Model file for the job. Use its own axes, mm. A direction names the side the tool comes from. Give positions to 0.01 mm unless a question says otherwise; leave off trailing zeros. Loops run counter-clockwise (first coordinate to the right, second up) from the corner with the lowest first, then second, coordinate; pieces in that order, holes last. Notation, with made-up numbers: (29.5, -19) - (87.5, -19) arc R5 cw to (87.5, -15) - close; hole circle Ø9 at (33.5, -8). An arc over 180 degrees is marked (long way). Use a Markdown table: item, result.
from build123d import *

# Parameters (mm, degrees)
SKETCH2_W           = 25
SKETCH2_H           = 25
BOSS_EXTRUDE1_DEPTH = 8
SKETCH5_R           = 0.7
CUT_EXTRUDE2_DEPTH  = 8
SKETCH2_6_W         = 25
SKETCH2_6_H         = 25
SKETCH2_6_W_2       = 20
SKETCH2_6_H_2       = 20
BOSS_EXTRUDE2_DEPTH = 43


with BuildPart() as part:
    # Sketch2 → Boss-Extrude1 (new body)
    with BuildSketch(Plane.XY.offset(43)):
        Rectangle(SKETCH2_W, SKETCH2_H)
    extrude(amount=BOSS_EXTRUDE1_DEPTH)

    # Sketch5 → Cut-Extrude2 (cut)
    with BuildSketch(Plane.XY.offset(43)):
        with Locations((-8.388056057, 8.509622087)):
            Circle(SKETCH5_R)
        with Locations((-6.038056057, 8.509622087)):
            Circle(SKETCH5_R)
        with Locations((-3.688056057, 8.509622087)):
            Circle(SKETCH5_R)
        with Locations((-1.338056057, 8.509622087)):
            Circle(SKETCH5_R)
        with Locations((1.011943943, 8.509622087)):
            Circle(SKETCH5_R)
        with Locations((3.361943943, 8.509622087)):
            Circle(SKETCH5_R)
        with Locations((5.711943943, 8.509622087)):
            Circle(SKETCH5_R)
        with Locations((8.061943943, 8.509622087)):
            Circle(SKETCH5_R)
        with Locations((-6.038056057, 6.159622087)):
            Circle(SKETCH5_R)
        with Locations((-3.688056057, 6.159622087)):
            Circle(SKETCH5_R)
        with Locations((-1.338056057, 6.159622087)):
            Circle(SKETCH5_R)
        with Locations((1.011943943, 6.159622087)):
            Circle(SKETCH5_R)
        with Locations((3.361943943, 6.159622087)):
            Circle(SKETCH5_R)
        with Locations((5.711943943, 6.159622087)):
            Circle(SKETCH5_R)
        with Locations((8.061943943, 6.159622087)):
            Circle(SKETCH5_R)
        with Locations((-6.038056057, 3.809622087)):
            Circle(SKETCH5_R)
        with Locations((-3.688056057, 3.809622087)):
            Circle(SKETCH5_R)
        with Locations((-1.338056057, 3.809622087)):
            Circle(SKETCH5_R)
        with Locations((1.011943943, 3.809622087)):
            Circle(SKETCH5_R)
        with Locations((3.361943943, 3.809622087)):
            Circle(SKETCH5_R)
        with Locations((5.711943943, 3.809622087)):
            Circle(SKETCH5_R)
        with Locations((8.061943943, 3.809622087)):
            Circle(SKETCH5_R)
        with Locations((-6.038056057, 1.459622087)):
            Circle(SKETCH5_R)
        with Locations((-3.688056057, 1.459622087)):
            Circle(SKETCH5_R)
        with Locations((-1.338056057, 1.459622087)):
            Circle(SKETCH5_R)
        with Locations((1.011943943, 1.459622087)):
            Circle(SKETCH5_R)
        with Locations((3.361943943, 1.459622087)):
            Circle(SKETCH5_R)
        with Locations((5.711943943, 1.459622087)):
            Circle(SKETCH5_R)
        with Locations((8.061943943, 1.459622087)):
            Circle(SKETCH5_R)
        with Locations((-6.038056057, -0.890377913)):
            Circle(SKETCH5_R)
        with Locations((-3.688056057, -0.890377913)):
            Circle(SKETCH5_R)
        with Locations((-1.338056057, -0.890377913)):
            Circle(SKETCH5_R)
        with Locations((1.011943943, -0.890377913)):
            Circle(SKETCH5_R)
        with Locations((3.361943943, -0.890377913)):
            Circle(SKETCH5_R)
        with Locations((5.711943943, -0.890377913)):
            Circle(SKETCH5_R)
        with Locations((8.061943943, -0.890377913)):
            Circle(SKETCH5_R)
        with Locations((-6.038056057, -3.240377913)):
            Circle(SKETCH5_R)
        with Locations((-3.688056057, -3.240377913)):
            Circle(SKETCH5_R)
        with Locations((-1.338056057, -3.240377913)):
            Circle(SKETCH5_R)
        with Locations((1.011943943, -3.240377913)):
            Circle(SKETCH5_R)
        with Locations((3.361943943, -3.240377913)):
            Circle(SKETCH5_R)
        with Locations((5.711943943, -3.240377913)):
            Circle(SKETCH5_R)
        with Locations((8.061943943, -3.240377913)):
            Circle(SKETCH5_R)
        with Locations((-6.038056057, -5.590377913)):
            Circle(SKETCH5_R)
        with Locations((-3.688056057, -5.590377913)):
            Circle(SKETCH5_R)
        with Locations((-1.338056057, -5.590377913)):
            Circle(SKETCH5_R)
        with Locations((1.011943943, -5.590377913)):
            Circle(SKETCH5_R)
        with Locations((3.361943943, -5.590377913)):
            Circle(SKETCH5_R)
        with Locations((5.711943943, -5.590377913)):
            Circle(SKETCH5_R)
        with Locations((8.061943943, -5.590377913)):
            Circle(SKETCH5_R)
        with Locations((-6.038056057, -7.940377913)):
            Circle(SKETCH5_R)
        with Locations((-3.688056057, -7.940377913)):
            Circle(SKETCH5_R)
        with Locations((-1.338056057, -7.940377913)):
            Circle(SKETCH5_R)
        with Locations((1.011943943, -7.940377913)):
            Circle(SKETCH5_R)
        with Locations((3.361943943, -7.940377913)):
            Circle(SKETCH5_R)
        with Locations((5.711943943, -7.940377913)):
            Circle(SKETCH5_R)
        with Locations((8.061943943, -7.940377913)):
            Circle(SKETCH5_R)
        with Locations((-8.388056057, 6.159622087)):
            Circle(SKETCH5_R)
        with Locations((-8.388056057, 3.809622087)):
            Circle(SKETCH5_R)
        with Locations((-8.388056057, 1.459622087)):
            Circle(SKETCH5_R)
        with Locations((-8.388056057, -0.890377913)):
            Circle(SKETCH5_R)
        with Locations((-8.388056057, -3.240377913)):
            Circle(SKETCH5_R)
        with Locations((-8.388056057, -5.590377913)):
            Circle(SKETCH5_R)
        with Locations((-8.388056057, -7.940377913)):
            Circle(SKETCH5_R)
    extrude(amount=CUT_EXTRUDE2_DEPTH, mode=Mode.SUBTRACT)

    # Sketch2<6> → Boss-Extrude2 (add)
    with BuildSketch(Plane.XY.offset(43)):
        Rectangle(SKETCH2_6_W, SKETCH2_6_H)
        Rectangle(SKETCH2_6_W_2, SKETCH2_6_H_2, mode=Mode.SUBTRACT)
    extrude(amount=-BOSS_EXTRUDE2_DEPTH)


solid = part.part
(1) Pin check, flat tips, straight feed: P1, Ø1.3, axis at x = -3.69, y = 8.51, coming from the +Z side; P2, Ø12, axis at x = 0.5, y = -2, coming from the -Z side. Stop position of each tip, or through.
Computed:
| item | result |
|---|---|
| P1 | through |
| P2 | z = 43 |
(2) Slice it at A-A, the plane z = 24.5. Write the cut outline in (x, y).
Computed:
| item | result |
|---|---|
| outline | (-12.5, -12.5) - (12.5, -12.5) - (12.5, 12.5) - (-12.5, 12.5) - close; hole (-10, -10) - (10, -10) - (10, 10) - (-10, 10) - close |
(3) Drill centre lines: probe 1 along X at (y, z) = (6.75, 22); probe 2 along Z at (x, y) = (4.25, 2.25). Where is each one in solid material? Low to high. Write a range as [from, to].
Computed:
| item | result |
|---|---|
| probe 1 | [-12.5, -10], [10, 12.5] |
| probe 2 | [43, 51] |
(4) Mould opens along Y. For faces 3 (the flat face through (0, 12.5, 26)), 4 (the cylindrical face through (-4.24, -3.67, 46.94)), 5 (the flat face through (0, 0, 51)) say: pulls with the +Y half, pulls with the -Y half, needs draft (parallel to the pull), parting line crosses it, or undercut.
Computed:
| item | result |
|---|---|
| face 3 | pulls with the +Y half |
| face 4 | undercut |
| face 5 | needs draft |
(5) 3-axis set-ups, long thin cutter, end or side, ignore diameter. For faces 1 (the cylindrical face through (0.86, 5.476, 46.944)), 2 (the flat face through (0, 0, 43)): which of +Z, -Z, +X, -X, +Y, -Y reach the whole face in a straight line?
Computed:
| item | result |
|---|---|
| face 1 | +Z, -Z |
| face 2 | -Z |
(6) Slice it at B-B, the plane x = 3.25. Count the separate pieces of the cut face and the enclosed holes in it, plus the area to 3 significant figures.
Computed:
| item | result |
|---|---|
| separate pieces | 9 |
| enclosed holes | 0 |
| area | 327 mm² |
